Autodesk Inventor part; units mm, degrees
ref_plane "f_XY" through (22.225, 0, 0) normal (0, 0, 1) x (1, 0, 0)
ref_plane "f_YZ" through (22.225, 0, 0) normal (1, 0, 0) x (0, 1, 0)
ref_plane "f_ZX" through (22.225, 0, 0) normal (0, 1, 0) x (0, 0, 1)
sketch "Sketch_18" plane through (0, 0, 0) normal (0, 0, 1) x (1, 0, 0)
  line L0 (22.225, 0) -> (0, 0)
  line L1 (0, 0) -> (0, 18.434)
  line L2 (0, 18.434) -> (0.762, 19.196)
  line L3 (0.762, 19.196) -> (4.318, 19.196)
  line L4 (4.318, 19.196) -> (5.334, 18.1801)
  line L5 (5.334, 18.1801) -> (6.35, 18.1801)
  line L6 (6.35, 18.1801) -> (6.35, 19.7675)
  line L7 (6.35, 19.7675) -> (21.463, 19.7675)
  line L8 (21.463, 19.7675) -> (22.225, 19.0055)
  line L9 (22.225, 19.0055) -> (22.225, 0)
  line L10 (22.225, 0) -> (0, 0)
revolve "Revolution1" add sketch "Sketch_18" angle 360 about axis through (22.225, 0, 0) along (1, 0, 0)
sketch "Sketch_21" plane through (0, 0, 0) normal (0, 0, 1) x (1, 0, 0)
  line L0 (44.45, 0) -> (22.225, 0)
  line L1 (22.225, 0) -> (22.225, 12.7)
  line L2 (22.225, 12.7) -> (42.926, 12.7)
  line L3 (42.926, 12.7) -> (44.45, 11.176)
  line L4 (44.45, 11.176) -> (44.45, 0)
  line L5 (44.45, 0) -> (22.225, 0)
revolve "Revolution2" add sketch "Sketch_21" angle 360 about axis through (44.45, 0, 0) along (1, 0, 0)
sketch "Sketch_9" plane through (44.45, 0, 0) normal (1, 0, 0) x (0, 0, -1)
  line L0 (-39.5351, -79.0702) -> (39.5351, -79.0702)
  line L1 (39.5351, -79.0702) -> (39.5351, 79.0702)
  line L2 (39.5351, 79.0702) -> (-39.5351, 79.0702)
  line L3 (-39.5351, 79.0702) -> (-39.5351, -79.0702)
  line L4 (-7.8359, -39.5351) -> (7.8359, -39.5351)
  line L5 (7.8359, -39.5351) -> (7.8359, 39.5351)
  line L6 (7.8359, 39.5351) -> (-7.8359, 39.5351)
  line L7 (-7.8359, 39.5351) -> (-7.8359, -39.5351)
extrude "Extrusion1" cut sketch "Sketch_9" against normal blind 22.225
sketch "Sketch4" plane through (0, 0, 0) normal (-1, 0, 0) x (0, 0, 1)
  point P0 (0, 0)
hole "Hole1" at (0, 0, 0) direction (1, 0, 0) diameter 13.5128 depth 20.4521 tip angle 120
sketch "Sketch_68" plane through (0, 0, 0) normal (0, 0.9998477, 0.0174524) x (1, 0, 0)
  line L0 (14.2748, -19.7675) -> (14.2748, 0)
  line L1 (14.2748, 0) -> (18.8978, 0)
  line L2 (18.8978, 0) -> (18.8978, -12.8333)
  line L3 (18.8978, -12.8333) -> (19.1143, -19.7675)
  line L4 (19.1143, -19.7675) -> (14.2748, -19.7675)
  line L5 (14.2748, -19.7675) -> (14.2748, 0)
revolve "Revolution3" cut sketch "Sketch_68" angle 360 about axis through (14.2748, -0.345, 19.7645) along (0, -0.0174524, 0.9998477)
thread "Thread1"
sketch "Sketch_20" plane through (0, 0, 0) normal (0, 0, 1) x (1, 0, 0)
  line L0 (6.35, 0) -> (0, 0)
  line L1 (0, 0) -> (0, 12.3063)
  line L2 (0, 12.3063) -> (6.35, 12.3063)
  line L3 (6.35, 12.3063) -> (6.35, 0)
  line L4 (6.35, 0) -> (0, 0)
revolve "Revolution4" cut sketch "Sketch_20" angle 360 about axis through (6.35, 0, 0) along (1, 0, 0)
sketch "Sketch_24" plane through (0, 0, 0) normal (0, 0, 1) x (1, 0, 0)
  line L0 (6.35, 0) -> (5.334, 0)
  line L1 (5.2675, 19.7675) -> (5.2675, 19.6834)
  line L2 (5.2675, 19.6834) -> (6.2166, 18.7343)
  arc A0 (6.2166, 18.5547) -> (6.2166, 18.7343) centre (6.1268, 18.6445) ccw
  line L3 (6.2166, 18.5547) -> (5.842, 18.1801)
  line L4 (5.842, 18.1801) -> (5.334, 18.1801)
  line L5 (5.334, 18.1801) -> (5.334, 17.9261)
  line L6 (5.334, 17.9261) -> (6.35, 17.9261)
  line L7 (6.35, 17.9261) -> (6.35, 18.8883)
  line L8 (6.35, 18.8883) -> (5.4707, 19.7675)
  line L9 (5.4707, 19.7675) -> (5.2675, 19.7675)
revolve "Revolution5" add sketch "Sketch_24" angle 360 about axis through (6.35, 0, 0) along (1, 0, 0)
sketch "Sketch_43" plane through (0, 0, 0) normal (0, 0, 1) x (1, 0, 0)
  circle A0 centre (34.925, 0) radius 4.7942
extrude "Extrusion2" cut sketch "Sketch_43" along normal mid plane 23.5077
ref_plane "f_XY" through (22.225, 0, 0) normal (0, 0, 1) x (1, 0, 0)
ref_plane "f_YZ" through (22.225, 0, 0) normal (1, 0, 0) x (0, 1, 0)
ref_plane "f_ZX" through (22.225, 0, 0) normal (0, 1, 0) x (0, 0, 1)
ref_plane "lovra1_XY" through (38.1, 0, 0) normal (1, 0, 0) x (0, 0, -1)
ref_plane "lovra1_YZ" through (38.1, 0, 0) normal (0, 0, -1) x (0, 1, 0)
ref_plane "lovra1_ZX" through (38.1, 0, 0) normal (0, 1, 0) x (1, 0, 0)
ref_plane "lovra2_XY" through (38.1, 11.049, 0) normal (1, 0, 0) x (0, 0, -1)
ref_plane "lovra2_YZ" through (38.1, 11.049, 0) normal (0, 0, -1) x (0, 1, 0)
ref_plane "lovra2_ZX" through (38.1, 11.049, 0) normal (0, 1, 0) x (1, 0, 0)
ref_plane "lovra21_XY" through (0, 0, 5.2705) normal (1, 0, 0) x (0, 0, -1)
ref_plane "lovra21_YZ" through (0, 0, 5.2705) normal (0, 0, -1) x (0, 1, 0)
ref_plane "lovra21_ZX" through (0, 0, 5.2705) normal (0, 1, 0) x (1, 0, 0)
ref_plane "lovra22_XY" through (0, 0, -5.2705) normal (1, 0, 0) x (0, 0, -1)
ref_plane "lovra22_YZ" through (0, 0, -5.2705) normal (0, 0, -1) x (0, 1, 0)
ref_plane "lovra22_ZX" through (0, 0, -5.2705) normal (0, 1, 0) x (1, 0, 0)
ref_plane "lovra3_XY" through (38.1, -11.049, 0) normal (1, 0, 0) x (0, 0, -1)
ref_plane "lovra3_YZ" through (38.1, -11.049, 0) normal (0, 0, -1) x (0, 1, 0)
ref_plane "lovra3_ZX" through (38.1, -11.049, 0) normal (0, 1, 0) x (1, 0, 0)
ref_plane "olen_XY" through (34.925, 0, 0) normal (1, 0, 0) x (0, 0, -1)
ref_plane "olen_YZ" through (34.925, 0, 0) normal (0, 0, -1) x (0, 1, 0)
ref_plane "olen_ZX" through (34.925, 0, 0) normal (0, 1, 0) x (1, 0, 0)
ref_plane "p1_XY" through (44.45, 0, 7.8359) normal (1, 0, 0) x (0, 0, -1)
ref_plane "p1_YZ" through (44.45, 0, 7.8359) normal (0, 0, -1) x (0, 1, 0)
ref_plane "p1_ZX" through (44.45, 0, 7.8359) normal (0, 1, 0) x (1, 0, 0)
ref_plane "p2_XY" through (44.45, 0, -7.8359) normal (1, 0, 0) x (0, 0, -1)
ref_plane "p2_YZ" through (44.45, 0, -7.8359) normal (0, 0, -1) x (0, 1, 0)
ref_plane "p2_ZX" through (44.45, 0, -7.8359) normal (0, 1, 0) x (1, 0, 0)
ref_plane "port_XY" through (14.2748, 0, 0) normal (0, 0, 1) x (1, 0, 0)
ref_plane "port_YZ" through (14.2748, 0, 0) normal (1, 0, 0) x (0, 1, 0)
ref_plane "port_ZX" through (14.2748, 0, 0) normal (0, 1, 0) x (0, 0, 1)
ref_plane "port2_XY" through (44.45, 0, 0) normal (1, 0, 0) x (0, 0, -1)
ref_plane "port2_YZ" through (44.45, 0, 0) normal (0, 0, -1) x (0, 1, 0)
ref_plane "port2_ZX" through (44.45, 0, 0) normal (0, 1, 0) x (1, 0, 0)
ref_plane "thd1_XY" through (44.45, 0, 0) normal (1, 0, 0) x (0, 0, -1)
ref_plane "thd1_YZ" through (44.45, 0, 0) normal (0, 0, -1) x (0, 1, 0)
ref_plane "thd1_ZX" through (44.45, 0, 0) normal (0, 1, 0) x (1, 0, 0)
ref_plane "thd2_XY" through (44.45, 0, 0) normal (1, 0, 0) x (0, 0, -1)
ref_plane "thd2_YZ" through (44.45, 0, 0) normal (0, 0, -1) x (0, 1, 0)
ref_plane "thd2_ZX" through (44.45, 0, 0) normal (0, 1, 0) x (1, 0, 0)
ref_plane "to_mounting_bracket_XY" through (22.225, 0, 0) normal (1, 0, 0) x (0, 0, -1)
ref_plane "to_mounting_bracket_YZ" through (22.225, 0, 0) normal (0, 0, -1) x (0, 1, 0)
ref_plane "to_mounting_bracket_ZX" through (22.225, 0, 0) normal (0, 1, 0) x (1, 0, 0)
ref_plane "to_nut_XY" through (0, 0, 0) normal (1, 0, 0) x (0, 0, -1)
ref_plane "to_nut_YZ" through (0, 0, 0) normal (0, 0, -1) x (0, 1, 0)
ref_plane "to_nut_ZX" through (0, 0, 0) normal (0, 1, 0) x (1, 0, 0)
ref_plane "to_pin_XY" through (34.925, 0, 0) normal (0, 0, 1) x (1, 0, 0)
ref_plane "to_pin_YZ" through (34.925, 0, 0) normal (1, 0, 0) x (0, 1, 0)
ref_plane "to_pin_ZX" through (34.925, 0, 0) normal (0, 1, 0) x (0, 0, 1)
ref_plane "to_screw_XY" through (14.2748, 14.2875, -10.0838) normal (0, 1, 0) x (1, 0, 0)
ref_plane "to_screw_YZ" through (14.2748, 14.2875, -10.0838) normal (1, 0, 0) x (0, 0, -1)
ref_plane "to_screw_ZX" through (14.2748, 14.2875, -10.0838) normal (0, 0, -1) x (0, 1, 0)
ref_plane "to_tube_XY" through (5.334, 0, 0) normal (1, 0, 0) x (0, 0, -1)
ref_plane "to_tube_YZ" through (5.334, 0, 0) normal (0, 0, -1) x (0, 1, 0)
ref_plane "to_tube_ZX" through (5.334, 0, 0) normal (0, 1, 0) x (1, 0, 0)
properties part number "17P0000_rear_head"
Work out the finished part from the listing and answer in its coordinate system (mm). A direction names the side the tool comes from. Give positions to 0.01 mm unless a question says otherwise; leave off trailing zeros. Loops run counter-clockwise (first coordinate to the right, second up) from the corner with the lowest first, then second, coordinate; pieces in that order, holes last. Notation, with made-up numbers: M 71,73.5 L 94,73.5 A24 ccw 94,112.5 Z; hole C 8.5,83 d1. An arc over 180 degrees is marked long. Use CSV: the item, a comma, the result in double quotes.
1) Find section A-A on x = 23.5. Write down the section's boundary in (y, z), plus the area to 3 significant figures.
Answer:
outline,"M -9.99,-7.84 L 9.99,-7.84 A12.7 ccw 9.99,7.84 L -9.99,7.84 A12.7 ccw Z; hole C 0,0 d2.95"
area,"364 mm^2"
2) Determine the mould class of faces 5 (the cylindrical face through (32.7, -12.7, 0.1)), 6 (the cylindrical face through (13.5, -0.3, -6.75)), 7 (the flat face through (44.45, 0, 0)) for opening direction Z: released by +Z, released by -Z, zero draft, split by the parting line, or undercut.
Answer:
face 5,"split by the parting line"
face 6,"undercut"
face 7,"zero draft"
3) Find section B-B on y = 2. Give the number of separate pieces and of enclosed holes in the cut face, plus the area to 3 significant figures.
Answer:
separate pieces,"3"
enclosed holes,"0"
area,"609 mm^2"
4) Which of the six approach directions +Z, -Z, +X, -X, +Y, -Y give full straight-line access (tool end or side, diameter ignored) to faces 1 (the cylindrical face through (32.7, 12.7, -0.1)), 2 (the conical face through (44.185, -11.44, -0.124)), 3 (the cylindrical face through (5.59, 17.34, 5.46)), 4 (the cylindrical face through (2.565, -2.499, 19.033))?
Answer:
face 1,"+X, +Y"
face 2,"+X, -Y"
face 3,"none"
face 4,"-X"
5) Consider L1, parallel to Z at x = 3, y = 0; L2, parallel to Y at x = 22, z = 1; L3, parallel to X at y = -5, z = -12.5 (3 decimals). Determine where each line is inside the solid, lowest interval first.
Answer:
L1,"-19.2 to -12.31, 12.31 to 19.2"
L2,"-19.2 to -3.95, 3.95 to 19.2"
L3,"0 to 22.225"
6) Given P1, Ø10, axis at x = 34.5, y = 2, coming from the -Z side; P2, Ø3, axis at x = 5.5, y = 14, coming from the +Z side; P3, Ø17.5, axis at y = 0, z = 0, coming from the -X side, each flat-ended and moving along its own axis, determine where each tip first touches the part or whether it passes through.
Answer:
P1,"z = -7.84"
P2,"z = 15.31"
P3,"x = 6.35"
